Source: CAD feature listing. Evaluate the final solid. Frame: model axes, mm. A direction names the side the tool comes from. Round coordinates to 2 decimals unless told otherwise and drop trailing zeros. Write each loop counter-clockwise with the first axis right and the second up, starting at its lowest first coordinate (ties: lowest second). Pieces come first, ordered by that corner, then holes.
from build123d import *

# Parameters (mm, degrees)
SKETCH1_R           = 2
BOSS_EXTRUDE1_DEPTH = 56
BOSS_EXTRUDE2_DEPTH = 2


with BuildPart() as part:
    # Sketch1 → Boss-Extrude1 (new body)
    with BuildSketch(Plane(origin=(0, 0, 0), x_dir=(1, 0, 0), z_dir=(0, 1, 0))):
        with Locations(Location((0, 0, 0), (0, 0, 270))):
            Circle(SKETCH1_R)
    extrude(amount=BOSS_EXTRUDE1_DEPTH)

    # Sketch2 → Boss-Extrude2 (add)
    with BuildSketch(Plane(origin=(0, 56, 0), x_dir=(1, 0, 0), z_dir=(0, 1, 0))):
        Polygon((2.039992028, -1.615670017), (2.419207293, 0.958849912), (0.379215264, 2.574519928), (-2.039992028, 1.615670017), (-2.419207293, -0.958849912), (-0.379215264, -2.574519928), align=None)
    extrude(amount=BOSS_EXTRUDE2_DEPTH)


solid = part.part
1) Reachability of faces 1 (the face through (-2, 28, 0)), 2 (the face through (2.227, 56.986, 0.346)) from +Z, -Z, +X, -X, +Y, -Y: full face, straight path, thin tool, end or side. Return the list, or none.
Taken from the geometry:
face 1: -Y
face 2: +Z, +X, +Y, -Y
2) Section query C-C on y = 12. Return the cut outline in (x, z).
Taken from the geometry:
outline: circle Ø4 at (0, 0)
3) Section query A-A on z = 0. Return the cut outline in (x, y).
Taken from the geometry:
outline: (-2.28, 56) - (-2, 56) - (-2, 0) - (2, 0) - (2, 56) - (2.28, 56) - (2.28, 58) - (-2.28, 58) - close
4) Contact query for flat-ended pins moving along their axis: P1, Ø1.5, axis at x = -2, z = 2, coming from the +Y side; P2, Ø1, axis at y = 50, z = 0.5, coming from the -X side. Output: stop coordinate, or through.
Taken from the geometry:
P1: stops at y = 58
P2: stops at x = -2
5) Material intervals for line 1 (Y direction, x = 1.9, z = -0.9); line 2 (X direction, y = 7, z = 1.65); line 3 (Z direction, x = 0.65, y = 31.5), sorted ascending.
Taken from the geometry:
line 1: y = 56 to 58
line 2: x = -1.13 to 1.13
line 3: z = -1.89 to 1.89
6) Section query B-B on x = -1.2. Return the cut outline in (y, z).
Taken from the geometry:
outline: (0, -1.6) - (56, -1.6) - (56, -1.95) - (58, -1.95) - (58, 1.92) - (56, 1.92) - (56, 1.6) - (0, 1.6) - close
